The model under review builds one solid part; all positions refer to its coordinate system, in mm. Face numbers are marked on the shaded views. A direction names the side the tool comes from. Round coordinates to 2 decimals unless told otherwise and drop trailing zeros. Loops run counter-clockwise (first coordinate to the right, second up) from the corner with the lowest first, then second, coordinate; pieces in that order, holes last. Notation, with made-up numbers: M 73.25,35.25 L 94.25,35.25 A21 ccw 94.25,72.25 Z; hole C -13.75,13.25 d10. An arc over 180 degrees is marked long. Answer in a Markdown table with one row per item. Add a question column.
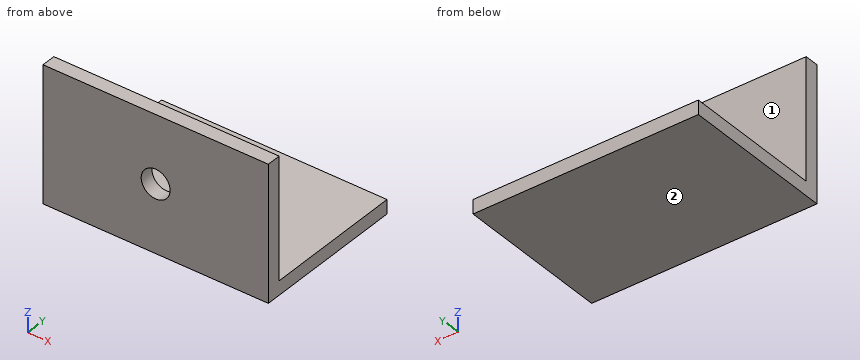
from build123d import *

# Parameters (mm, degrees)
SKETCH1_W           = 50.8
SKETCH1_H           = 30.48
BOSS_EXTRUDE1_DEPTH = 3.175
SKETCH2_W           = 50.8
SKETCH2_H           = 3.175
BOSS_EXTRUDE2_DEPTH = 31.75
SKETCH3_R           = 3.2639
CUT_EXTRUDE1_DEPTH  = 50.8


with BuildPart() as part:
    # Sketch1 → Boss-Extrude1 (new body)
    with BuildSketch(Plane(origin=(0, 0, 0), x_dir=(1, 0, 0), z_dir=(0, 1, 0))):
        Rectangle(SKETCH1_W, SKETCH1_H)
    extrude(amount=BOSS_EXTRUDE1_DEPTH)

    # Sketch2 → Boss-Extrude2 (add)
    with BuildSketch(Plane(origin=(0, 3.175, 0), x_dir=(1, 0, 0), z_dir=(0, 1, 0))):
        with Locations((0, 13.6525)):
            Rectangle(SKETCH2_W, SKETCH2_H)
    extrude(amount=BOSS_EXTRUDE2_DEPTH)

    # Sketch3 → Cut-Extrude1 (cut)
    with BuildSketch(Plane.XZ):
        Circle(SKETCH3_R)
    extrude(amount=-CUT_EXTRUDE1_DEPTH, mode=Mode.SUBTRACT)


solid = part.part
1. Take a section at A-A, the plane x = 0. State the section outline as (y, z) points (3 decimals).
2. Take a section at B-B, the plane z = 0. State the section outline as (x, y) points (3 decimals).
3. For pin 1 Ø16 at (x, y) = (-6, 14.5) entering from +Z (3 decimals); pin 2 Ø6 at (x, z) = (-13.5, -7) entering from +Y (3 decimals); pin 3 Ø5 at (x, z) = (0, 0) entering from -Y; pin 4 Ø1 at (x, z) = (-7.5, -8.5) entering from -Y, all flat-tipped, find the tip position at first contact; note any pin that passes through.
4. Machinability: for the marked faces 1 and 2, which of the approach directions +Z, -Z, +X, -X, +Y, -Y give a long, thin tool a straight path to every point of the face, cutting with its end or side? Answer none if there is none.
5. Take a section at D-D, the plane y = 32.5. State the section outline as (x, z) points (3 decimals), and give its area (3 significant figures).
6. Take a section at C-C, the plane x = 9.5. State the section outline as (y, z) points (3 decimals), and give its area (3 significant figures).
7. To check wall thickness, follow probe 1 along Z at (x, y) = (0, 1.85); probe 2 along Y at (x, z) = (-21.5, 0.5) (3 decimals); probe 3 along Z at (x, y) = (-1, 29.5) (3 decimals). State the ranges of each line that lie inside material, in increasing order.
Check sheet entries:
| question | item | result |
|---|---|---|
| 1 | outline | M 0,-15.24 L 34.925,-15.24 L 34.925,-12.065 L 3.175,-12.065 L 3.175,-3.264 L 0,-3.264 Z; M 0,3.264 L 3.175,3.264 L 3.175,15.24 L 0,15.24 Z |
| 2 | outline | M -25.4,0 L -3.264,0 L -3.264,3.175 L -25.4,3.175 Z; M 3.264,0 L 25.4,0 L 25.4,3.175 L 3.264,3.175 Z |
| 3 | pin 1 | stops at z = -12.065 |
| 3 | pin 2 | stops at y = 3.175 |
| 3 | pin 3 | passes through |
| 3 | pin 4 | stops at y = 0 |
| 4 | face 1 | +Z, +X, -X, +Y |
| 4 | face 2 | -Z, +X, -X, +Y, -Y |
| 5 | outline | M -25.4,-15.24 L 25.4,-15.24 L 25.4,-12.065 L -25.4,-12.065 Z |
| 5 | area | 161 mm^2 |
| 6 | outline | M 0,-15.24 L 34.925,-15.24 L 34.925,-12.065 L 3.175,-12.065 L 3.175,15.24 L 0,15.24 Z |
| 6 | area | 198 mm^2 |
| 7 | probe 1 | z = -15.24 to -3.26, 3.26 to 15.24 |
| 7 | probe 2 | y = 0 to 3.175 |
| 7 | probe 3 | z = -15.24 to -12.065 |
